Design review of the part built by this model. Coordinates are the model's own, in mm. A direction names the side the tool comes from. Coordinates: 2 decimals unless noted, no trailing zeros. Loops run counter-clockwise (first coordinate to the right, second up) from the corner with the lowest first, then second, coordinate; pieces in that order, holes last. Notation, with made-up numbers: (16.25, -23) -> (34.25, -23) arc R29 ccw to (34.25, 11) -> close; hole circle Ø2 at (14, 65). An arc over 180 degrees is marked (long way). Answer in a Markdown table with one row per item.
```python
from build123d import *

# Parameters (mm, degrees)
F0_W     = 20
F0_H     = 20
F0_R     = 3
F1_DEPTH = 5
F0_W_2   = 10
F2_DEPTH = 25
F3_R     = 3
F4_DEPTH = 25


# Not quite as in the source:
# - a feature names something its author has since deleted; it is built from what else it names


with BuildPart() as f1:
    # F0 (on Top) → F1 (new body)
    with BuildSketch(Plane.XY):
        with Locations((20, 10)):
            Rectangle(F0_W, F0_H)
        with Locations((20, 10)):
            Circle(F0_R, mode=Mode.SUBTRACT)
    extrude(amount=F1_DEPTH)

    # F0 (on Top) → F2 (join)
    with BuildSketch(Plane.XY):
        with Locations((5, 10)):
            Rectangle(F0_W_2, F0_H)
    extrude(amount=F2_DEPTH)

    # F3 (on Right) → F4 (cut)
    with BuildSketch(Plane.YZ):
        with Locations((10, 14)):
            Circle(F3_R)
    extrude(amount=F4_DEPTH, mode=Mode.SUBTRACT)


solid = f1.part
```
(1) Draft analysis for pull direction X (two halves, no side actions). For faces 3 (the cylindrical face through (17, 10, 2)), 4 (the cylindrical face through (4.93, 11.384, 11.338)), 5 (the flat face through (0, 10, 10)), state which applies: pulls with the +X half, pulls with the -X half, needs draft (parallel to the pull), parting line crosses it, or undercut.
Evaluation:
| item | result |
|---|---|
| face 3 | undercut |
| face 4 | needs draft |
| face 5 | pulls with the -X half |
(2) Take a section at D-D on z = 2. Give the boundary of the cut face in (x, y), and give its area (3 significant figures).
Evaluation:
| item | result |
|---|---|
| outline | (0, 0) -> (30, 0) -> (30, 20) -> (0, 20) -> close; hole circle Ø6 at (20, 10) |
| area | 572 mm² |
(3) Take a section at C-C on x = 20. Give the boundary of the cut face in (y, z), and give its area (3 significant figures).
Evaluation:
| item | result |
|---|---|
| outline | (0, 0) -> (7, 0) -> (7, 5) -> (0, 5) -> close; (13, 0) -> (20, 0) -> (20, 5) -> (13, 5) -> close |
| area | 70.0 mm² |
(4) For pin 1 (9.5 mm diameter, centred on y = 10, z = 14, fed in from +X); pin 2 (9.5 mm diameter, centred on x = 20, y = 10, fed in from +Z); pin 3 (10 mm diameter, centred on x = 17, z = 14, fed in from +Y), all flat-tipped, find the tip position at first contact; note any pin that passes through.
Evaluation:
| item | result |
|---|---|
| pin 1 | stops at x = 10 |
| pin 2 | stops at z = 5 |
| pin 3 | passes through |
(5) Take a section at B-B on z = 14. Give the boundary of the cut face in (x, y), and give its area (3 significant figures).
Evaluation:
| item | result |
|---|---|
| outline | (0, 0) -> (10, 0) -> (10, 7) -> (0, 7) -> close; (0, 13) -> (10, 13) -> (10, 20) -> (0, 20) -> close |
| area | 140 mm² |
(6) Tool access review of faces 1 (the flat face through (10, 12, 17)), 2 (the flat face through (5, 10, 25)): name each direction out of +Z, -Z, +X, -X, +Y, -Y from which nothing blocks a thin tool from reaching the whole face with its end or side.
Evaluation:
| item | result |
|---|---|
| face 1 | +Z, +X, +Y, -Y |
| face 2 | +Z, +X, -X, +Y, -Y |
(7) To check wall thickness, follow probe 1 along Y at (x, z) = (7.75, 14); probe 2 along Z at (x, y) = (2, 10); probe 3 along Z at (x, y) = (13.5, 1.75). State the ranges of each line that lie inside material, in increasing order.
Evaluation:
| item | result |
|---|---|
| probe 1 | y = 0 to 7, 13 to 20 |
| probe 2 | z = 0 to 11, 17 to 25 |
| probe 3 | z = 0 to 5 |
(8) Take a section at A-A on y = 10. Give the boundary of the cut face in (x, z), and give its area (3 significant figures).
Evaluation:
| item | result |
|---|---|
| outline | (0, 0) -> (17, 0) -> (17, 5) -> (10, 5) -> (10, 11) -> (0, 11) -> close; (0, 17) -> (10, 17) -> (10, 25) -> (0, 25) -> close; (23, 0) -> (30, 0) -> (30, 5) -> (23, 5) -> close |
| area | 260 mm² |
